```python
from build123d import *

# Parameters (mm, degrees)
SKETCH_1_R        = 5.5
EXTRUDE_311_DEPTH = 9
SKETCH_2_R        = 0.75
EXTRUDE_525_DEPTH = 10


with BuildPart() as part:
    # Эскиз1 → Extrude 311 (new, symmetric)
    with BuildSketch(Plane.XY):
        Circle(SKETCH_1_R)
    extrude(amount=EXTRUDE_311_DEPTH, both=True)

    # Эскиз2 → Extrude 525 (add)
    with BuildSketch(Plane.XY.offset(9)):
        with Locations((0, -0.775)):
            Circle(SKETCH_2_R)
        with Locations((0, 0.775)):
            Circle(SKETCH_2_R)
    extrude(amount=EXTRUDE_525_DEPTH)


solid = part.part
```
Work out the finished part from the listing and answer in its coordinate system (mm). A direction names the side the tool comes from. Give positions to 0.01 mm unless a question says otherwise; leave off trailing zeros. Write each loop counter-clockwise with the first axis right and the second up, starting at its lowest first coordinate (ties: lowest second). Pieces come first, ordered by that corner, then holes. Notation, with made-up numbers: (85.5, 60.25) -> (119.5, 60.25) arc R28 ccw to (119.5, 81.25) -> close; hole circle Ø4 at (-8.5, -14.75). An arc over 180 degrees is marked (long way). Write item = value, one per line.
Q1. Section B-B on z = 16 is taken. Determine the outline of the cut face in (x, y) (3 decimals), and give its area (3 significant figures).
Computed values:
outline = circle Ø1.5 at (0, -0.775); circle Ø1.5 at (0, 0.775)
area = 3.53 mm^2
Q2. Section D-D on z = 8 is taken. Determine the outline of the cut face in (x, y).
Computed values:
outline = circle Ø11 at (0, 0)
Q3. Section A-A on x = 0 is taken. Determine the outline of the cut face in (y, z) (3 decimals).
Computed values:
outline = (-5.5, -9) -> (5.5, -9) -> (5.5, 9) -> (1.525, 9) -> (1.525, 19) -> (0.025, 19) -> (0.025, 9) -> (-0.025, 9) -> (-0.025, 19) -> (-1.525, 19) -> (-1.525, 9) -> (-5.5, 9) -> close
Q4. Section C-C on y = 1.25 is taken. Determine the outline of the cut face in (x, z).
Computed values:
outline = (-5.36, -9) -> (5.36, -9) -> (5.36, 9) -> (0.58, 9) -> (0.58, 19) -> (-0.58, 19) -> (-0.58, 9) -> (-5.36, 9) -> close
Q5. Consider line 1 along Z through (x, y) = (1.5, -1); line 2 along X through (y, z) = (4.75, 5.75); line 3 along X through (y, z) = (-1.5, -0.25). Determine where each line is inside the solid, lowest interval first.
Computed values:
line_1 = -9 to 9
line_2 = -2.77 to 2.77
line_3 = -5.29 to 5.29
Q6. For a pull along Y with two mould halves and no side action, classify faces 1 (the flat face through (0, -1, 19)), 2 (the cylindrical face through (-0.75, 0.81, 13.93)), 3 (the cylindrical face through (-1.19, -5.37, 0.13)) as pulls with the +Y half, pulls with the -Y half, needs draft (parallel to the pull), parting line crosses it, or undercut.
Computed values:
face_1 = needs draft
face_2 = undercut
face_3 = parting line crosses it
Q7. A tool of negligible diameter and unlimited length cuts with its end or side. For faces 4 (the cylindrical face through (-0.75, -0.74, 13.93)), 5 (the flat face through (0, 1, 19)), from which of +Z, -Z, +X, -X, +Y, -Y can it reach the whole face along a straight path? Write none if from no direction.
Computed values:
face_4 = +Z
face_5 = +Z, +X, -X, +Y, -Y
Q8. Flat-ended cylindrical pins translate along their axes: pin 1 Ø1.5 at (x, y) = (-1, 2.5) entering from +Z; pin 2 Ø2 at (y, z) = (2.5, 6.5) entering from -X. Find the tip coordinate at first contact, or state that the pin passes through.
Computed values:
pin_1 = 9
pin_2 = -5.29
